Source: three-view drawing plus pictorial views. Frame: mm from the lowest corner of the part. Give positions to 0.01 mm unless a question says otherwise; leave off trailing zeros. Order: outer loops, then holes, each group sorted by start corner. A loop starts at its lowest first (then second) coordinate and runs counter-clockwise, first axis right, second up.
1) Section A-A, the plane y = 2.2. Return loops of the section in (x, z).
2) Material intervals for line 1 (Z direction, x = 10, y = 2.05); line 2 (X direction, y = 0.7, z = 11.5); line 3 (Z direction, x = 5, y = 1.9), sorted ascending.
3) First-contact query: P1, Ø2.5, axis at x = 10, z = 72, coming from the +Y side; P2, Ø1, axis at x = 11.5, y = 1.5, coming from the +Z side. Flat tips, straight axial feed; report the tip coordinate or a pass-through.
4) Section B-B, the plane x = 5. Return loops of the section in (y, z), plus the area to 3 significant figures.
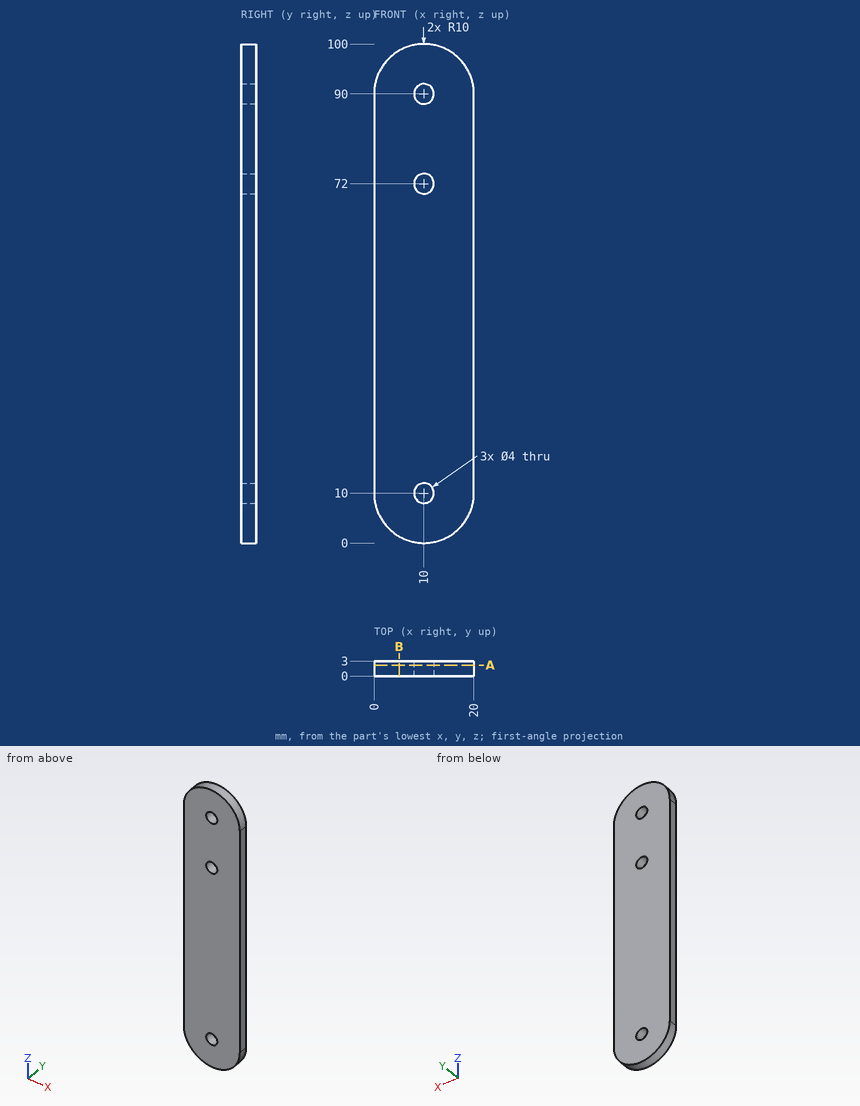
From the geometry:
1. outline: (0, 10) arc R10 ccw to (20, 10) - (20, 90) arc R10 ccw to (0, 90) - close; hole circle Ø4 at (10, 10); hole circle Ø4 at (10, 72); hole circle Ø4 at (10, 90)
2. line 1: z = 0 to 8, 12 to 70, 74 to 88, 92 to 100
2. line 2: x = 0 to 8.68, 11.32 to 20
2. line 3: z = 1.34 to 98.66
3. P1: passes through
3. P2: stops at z = 99.95
4. outline: (0, 1.34) - (3, 1.34) - (3, 98.66) - (0, 98.66) - close
4. area: 292 mm2
